```python
from build123d import *

# Parameters (mm, degrees)
EXTRUDE_1_DEPTH     = 76
EXTRUDE_2_DEPTH     = 2
CUT_EXTRUDE_1_DEPTH = 10
SKETCH_5_W          = 2
SKETCH_5_H          = 76
EXTRUDE_3_DEPTH     = 10


with BuildPart() as part:
    # 草图1 → 凸台-拉伸1 (new body)
    with BuildSketch(Plane.XY):
        Polygon((-92, 0), (0, 0), (0, 55.5), (-2, 55.5), (-2, 2), (-92, 2), align=None)
    extrude(amount=EXTRUDE_1_DEPTH)

    # 草图3 → 凸台-拉伸2 (add)
    with BuildSketch(Plane.XY.offset(76)):
        Polygon((0, 55.5), (-10, 55.5), (-10, 10), (-92, 10), (-92, 0), (0, 0), align=None)
    extrude(amount=EXTRUDE_2_DEPTH)

    # 草图4 → 切除-拉伸1 (cut)
    with BuildSketch(Plane.XZ):
        with BuildLine():
            Line((-87, 0), (-87, 32))
            ThreePointArc((-87, 32), (-46, 73), (-5, 32))
            Line((-5, 32), (-5, 0))
            Line((-5, 0), (-87, 0))
        make_face()
    extrude(amount=-CUT_EXTRUDE_1_DEPTH, mode=Mode.SUBTRACT)

    # 草图5 → 凸台-拉伸3 (add)
    with BuildSketch(Plane(origin=(0, 2, 0), x_dir=(1, 0, 0), z_dir=(0, 1, 0))):
        with Locations((-91, -38)):
            Rectangle(SKETCH_5_W, SKETCH_5_H)
    extrude(amount=EXTRUDE_3_DEPTH)


solid = part.part
```
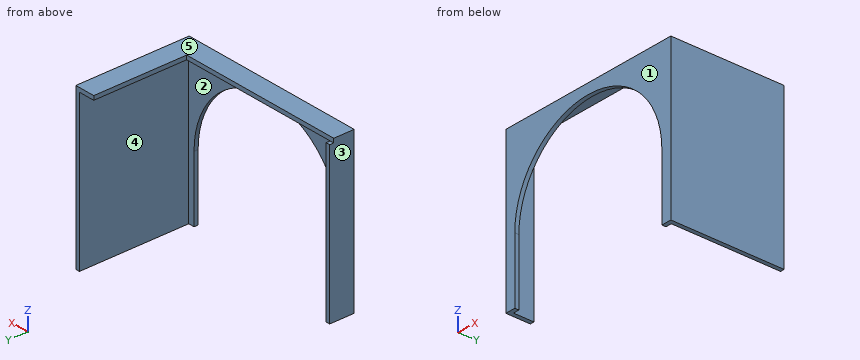
Design review of the part built by this model. Coordinates are the model's own, in mm. Face numbers are marked on the shaded views. A direction names the side the tool comes from. Coordinates: 2 decimals unless noted, no trailing zeros. Loops run counter-clockwise (first coordinate to the right, second up) from the corner with the lowest first, then second, coordinate; pieces in that order, holes last.
Q1. We need section A-A on z = 17.5. State the section outline as (x, y) points, and give its area (3 significant figures).
Reported:
outline: (-92, 0) - (-87, 0) - (-87, 2) - (-90, 2) - (-90, 12) - (-92, 12) - close; (-5, 0) - (0, 0) - (0, 55.5) - (-2, 55.5) - (-2, 2) - (-5, 2) - close
area: 147 mm2
Q2. We need section C-C on x = -46. State the section outline as (y, z) points.
Reported:
outline: (0, 73) - (2, 73) - (2, 76) - (10, 76) - (10, 78) - (0, 78) - close
Q3. We need section B-B on y = 52.5. State the section outline as (x, z) points.
Reported:
outline: (-10, 76) - (-2, 76) - (-2, 0) - (0, 0) - (0, 78) - (-10, 78) - close
Q4. The part is to be moulded in two halves that separate along X. For the marked faces 1, 2 and 3, say which applies: +X half, -X half, draft (parallel to the pull), parting line (faces both ways), or undercut.
Reported:
face 1: draft
face 2: undercut
face 3: -X half
Q5. To check wall thickness, follow line 1 (X direction, y = 8.5, z = 57); line 2 (Z direction, x = -75.5, y = 3); line 3 (X direction, y = 26.5, z = 58). State the ranges of each line that lie inside material, in increasing order.
Reported:
line 1: x = -92 to -90, -2 to 0
line 2: z = 76 to 78
line 3: x = -2 to 0
Q6. Tool access review of the marked faces 4 and 5: name each direction out of +Z, -Z, +X, -X, +Y, -Y from which nothing blocks a thin tool from reaching the whole face with its end or side.
Reported:
face 4: -Z, +Y
face 5: +Z, +X, -X, +Y, -Y
Q7. We need section D-D on z = 46. State the section outline as (x, y) points, and give its area (3 significant figures).
Reported:
outline: (-92, 0) - (-84.54, 0) - (-84.54, 2) - (-90, 2) - (-90, 12) - (-92, 12) - close; (-7.46, 0) - (0, 0) - (0, 55.5) - (-2, 55.5) - (-2, 2) - (-7.46, 2) - close
area: 157 mm2
Q8. For pin 1 (1.6 mm diameter, centred on x = -37, z = 77, fed in from +Y); pin 2 (0.6 mm diameter, centred on y = 1, z = 19, fed in from +X); pin 3 (1 mm diameter, centred on x = -90.5, z = 53, fed in from +Y); pin 4 (4 mm diameter, centred on y = 45.5, z = 33, fed in from -X), all flat-tipped, find the tip position at first contact; note any pin that passes through.
Reported:
pin 1: stops at y = 10
pin 2: stops at x = 0
pin 3: stops at y = 12
pin 4: stops at x = -2
